Here's how the part is built. I have some questions about the finished solid (model axes, mm). Face numbers are marked on the shaded views. Give positions to 0.01 mm unless a question says otherwise; leave off trailing zeros. Write each loop counter-clockwise with the first axis right and the second up, starting at its lowest first coordinate (ties: lowest second). Pieces come first, ordered by that corner, then holes. Notation, with made-up numbers: (3.5, 33.5) - (28.5, 33.5) arc R29 cw to (28.5, 63.5) - close; hole circle Ø11 at (70, -19). An arc over 180 degrees is marked (long way). One line per item, written item: value. Start each with the question number.
1) We'd pull the mould along X, two halves only. Please class the marked faces 1, 2 and 3: +X half, -X half, draft (parallel to the pull), parting line (faces both ways), or undercut.
2) I'm going to push flat-ended pins straight in: P1, Ø4, axis at y = -24.5, z = -31.5, coming from the +X side; P2, Ø4, axis at x = 31.5, y = -29.5, coming from the -Z side; P3, Ø12, axis at y = -16.5, z = -39.5, coming from the -X side. Where does each tip first touch, or does it pass through?
3) Imagine slicing it at A-A on y = -13.5. Write out the boundary of the cut face in (x, z) (3 decimals), plus the area to 3 significant figures.
4) Please list where these lines run through material, in increasing order: L1, parallel to X at y = -15.5, z = 27.5; L2, parallel to Z at x = -19, y = -8.5; L3, parallel to X at y = -30, z = 29. Write a range as [from, to].
from build123d import *

# Parameters (mm, degrees)
F1_DEPTH = 34.036
F2_R     = 9.4659800125
F3_DEPTH = 76.962
F4_R     = 5.08


with BuildPart() as f1:
    # F0 (on Front) → F1 (new body)
    with BuildSketch(Plane.XZ):
        Polygon((55.3876371372, -6.7820224733), (23.5658078206, 50.581013021), (-40.8231669317, 38.0428077057), (-48.7959125128, -27.0692648314), (10.6656344867, -54.772533422), align=None)
    extrude(amount=F1_DEPTH)

    # F2 (on face) → F3 (join)
    with BuildSketch(Plane(origin=(39.4767224789, 0, 21.8994952738), x_dir=(0, 1, 0), z_dir=(0.8744581925, 0, 0.4851008861))):
        with Locations((-16.4809413254, -6.0359826311)):
            Circle(F2_R)
    extrude(amount=F3_DEPTH)

    # F4
    f4_edges = [f1.edges().sort_by_distance(p)[0] for p in [
        (39.476722, 0, 21.899495),
        (55.387637, -17.018, -6.782022),
        (23.565808, -17.018, 50.581013),
        (39.476722, -34.036, 21.899495),
        (33.026636, -34.036, -30.777278),
        (10.665634, -17.018, -54.772533),
        (33.026636, 0, -30.777278),
        (-8.62868, 0, 44.31191),
        (-8.62868, -34.036, 44.31191),
        (-44.80954, -34.036, 5.486771),
        (-19.065139, -34.036, -40.920899),
        (-40.823167, -17.018, 38.042808),
        (-48.795913, -17.018, -27.069265),
        (-44.80954, 0, 5.486771),
        (-19.065139, 0, -40.920899),
    ]]
    fillet(f4_edges, radius=F4_R)


solid = f1.part
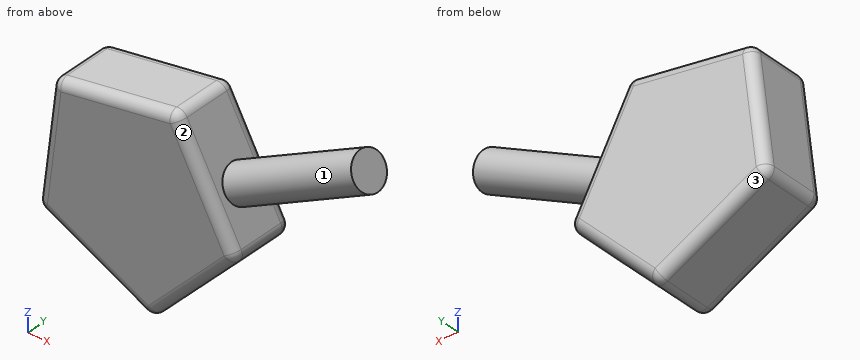
Numbers:
1. face 1: undercut
1. face 2: +X half
1. face 3: -X half
2. P1: x = 34.22
2. P2: z = -34.53
2. P3: x = -34.99
3. outline: (-48.347, -23.406) arc R5.08 ccw to (-45.45, -28.628) - (7.32, -53.214) arc R5.08 ccw to (13.182, -52.072) - (52.871, -9.482) arc R5.08 ccw to (53.597, -3.555) - (46.763, 8.765) - (114.063, 46.099) - (105.347, 61.812) - (38.046, 24.478) - (25.356, 47.354) arc R5.08 ccw to (19.943, 49.876) - (-37.2, 38.748) arc R5.08 ccw to (-41.272, 34.379) - close
3. area: 8,770 mm^2
4. L1: [-42.11, 36.37], [42.61, 81.42]
4. L2: [-40.95, 42.29]
4. L3: [-41.82, 35.41]
